Check sheet for the modelled part. Datum: model origin and axes. Units: mm. A direction names the side the tool comes from. Round coordinates to 2 decimals unless told otherwise and drop trailing zeros. Write each loop counter-clockwise with the first axis right and the second up, starting at its lowest first coordinate (ties: lowest second). Pieces come first, ordered by that corner, then holes. Notation, with made-up numbers: M 61.25,39.25 L 118.25,39.25 A28 cw 118.25,73.25 Z; hole C -32.5,56 d2. An arc over 180 degrees is marked long. Put each result on its own line as item: value.
```python
from build123d import *

# Parameters (mm, degrees)
BOSS_EXTRUDE1_DEPTH = 5
SKETCH3_OUTSIDE_W   = 23.682
SKETCH3_OUTSIDE_H   = 22.466
SKETCH3_OUTSIDE_R   = 3.931755333
CUT_EXTRUDE1_DEPTH  = 5
CUT_EXTRUDE1_DRAFT  = -45
BOSS_EXTRUDE2_DEPTH = 1
SKETCH5_R           = 3.56
BOSS_EXTRUDE3_DEPTH = 2.5
SKETCH6_R           = 2.5
CUT_EXTRUDE2_DEPTH  = 12.056672194


with BuildPart() as part:
    # Sketch2 → Boss-Extrude1 (new body)
    with BuildSketch(Plane(origin=(0, 0, 0), x_dir=(1, 0, 0), z_dir=(0, 1, 0))):
        Polygon((2.27, -3.931755333), (4.54, 0), (2.27, 3.931755333), (-2.27, 3.931755333), (-4.54, 0), (-2.27, -3.931755333), align=None)
    extrude(amount=BOSS_EXTRUDE1_DEPTH)


with BuildPart() as cut_extrude1_tool:
    # Sketch3 outside → Cut-Extrude1 (with draft: the straight prism first)
    with BuildSketch(Plane(origin=(0, 5, 0), x_dir=(1, 0, 0), z_dir=(0, 1, 0))):
        Rectangle(SKETCH3_OUTSIDE_W, SKETCH3_OUTSIDE_H)
        Circle(SKETCH3_OUTSIDE_R, mode=Mode.SUBTRACT)
    extrude(amount=-CUT_EXTRUDE1_DEPTH)
    # Cut-Extrude1: the draft: its side faces are tilted about the plane it starts from
    cut_extrude1_sides = [cut_extrude1_tool.faces().sort_by_distance(p)[0] for p in [
        (0, 2.5, 11.233),
        (11.841, 2.5, 0),
        (0, 2.5, -11.233),
        (-11.841, 2.5, 0),
        (-3.931755333, 2.5, 0),
    ]]
    draft(cut_extrude1_sides, Plane(origin=(0, 5, 0), x_dir=(1, 0, 0), z_dir=(0, 1, 0)), CUT_EXTRUDE1_DRAFT)


with BuildPart() as part_1:
    add(part.part)

    # Cut-Extrude1: cut by cut_extrude1_tool
    add(cut_extrude1_tool.part, mode=Mode.SUBTRACT)

    # Sketch4 → Boss-Extrude2 (add)
    with BuildSketch(Plane.XZ):
        with BuildLine():
            Line((-1.7, -4.702127178), (1.7, -4.702127178))
            ThreePointArc((1.7, -4.702127178), (0, 5), (-1.7, -4.702127178))
        make_face()
    extrude(amount=BOSS_EXTRUDE2_DEPTH)

    # Sketch5 → Boss-Extrude3 (add)
    with BuildSketch(Plane.XZ.offset(1)):
        with Locations(Location((0, 0, 0), (0, 0, 270))):
            Circle(SKETCH5_R)
    extrude(amount=BOSS_EXTRUDE3_DEPTH)

    # Sketch6 → Cut-Extrude2 (cut, through all)
    with BuildSketch(Plane.XZ.offset(3.5)):
        with Locations(Location((0, -0.79, 0), (0, 0, 270))):
            Circle(SKETCH6_R)
    extrude(amount=-CUT_EXTRUDE2_DEPTH, mode=Mode.SUBTRACT)


solid = part_1.part
```
1. Release check for a two-part mould opening along X. For faces 6 (the flat face through (0, 2, -3.932)), 7 (the flat face through (3.42, 2.46, -1.94)), 8 (the cylindrical face through (-2.44, 0.69, -0.25)), 9 (the flat face through (-3.42, 2.46, 1.94)) record: +X half, -X half, draft (parallel to the pull), parting line (faces both ways), or undercut.
Computed values:
face 6: draft
face 7: +X half
face 8: undercut
face 9: -X half
2. Cross-section at A-A (y = 3.75). Enter the section's corners in (x, z).
Computed values:
outline: M -4.54,0 L -2.27,-3.93 L 2.27,-3.93 L 4.54,0 L 2.27,3.93 L -2.27,3.93 Z; hole C 0,-0.79 d5
3. Scan lines: probe 1 along Y at (x, z) = (-4.5, -2); probe 2 along X at (y, z) = (1, -2.25); probe 3 along Z at (x, y) = (-0.5, 2.75). Record each from-to range of solid material in increasing order.
Computed values:
probe 1: y = -1 to 0
probe 2: x = -3.24 to -2.03, 2.03 to 3.24
probe 3: z = -3.93 to -3.24, 1.66 to 3.93
4. Depth check by flat-ended pin: pin 1 Ø5 at (y, z) = (-2, 3) entering from +X; pin 2 Ø3 at (x, y) = (0, 3.5) entering from -Z; pin 3 Ø3 at (x, z) = (0, -0.79) entering from +Y; pin 4 Ø1 at (x, z) = (4, 2.5) entering from +Y. Enter the tip coordinate at first touch or a pass-through.
Computed values:
pin 1: stops at x = 4.95
pin 2: stops at z = -3.93
pin 3: passes through
pin 4: stops at y = 0
5. Access from +Z, -Z, +X, -X, +Y, -Y to the whole of each face (thin tool, end or side, straight path). Record for faces 1 (the flat face through (-3.39, 2.46, -1.99)), 2 (the conical face through (-4.08, 4.85, -0.01)), 3 (the cylindrical face through (-2.2, -2.2, 2.8)), 4 (the flat face through (0, 2, 3.932)), 5 (the flat face through (3.39, 2.46, 1.99)).
Computed values:
face 1: -Z, -X, +Y
face 2: -X, +Y
face 3: -Y
face 4: +Z, +X, -X, +Y
face 5: +Z, +X, +Y
